Read the model definition and answer for the solid it produces. Units are mm, in the model's axes. Face numbers are marked on the shaded views. A direction names the side the tool comes from. Give positions to 0.01 mm unless a question says otherwise; leave off trailing zeros. Write each loop counter-clockwise with the first axis right and the second up, starting at its lowest first coordinate (ties: lowest second). Pieces come first, ordered by that corner, then holes.
```python
from build123d import *

# Parameters (mm, degrees)
SKETCH011_W         = 30
SKETCH011_H         = 50
PAD009_DEPTH        = 4
SKETCH007_W         = 50
SKETCH007_H         = 25
PAD006_DEPTH        = 4
PAD007_DEPTH        = 3
PAD005_DEPTH        = 1
PAD008_DEPTH        = 3
HOLE001_D           = 4.4
HOLE001_DEPTH       = 25
HOLE001_CSINK_D     = 8
HOLE001_CSINK_ANGLE = 90
SKETCH012_W         = 40.900608
SKETCH012_H         = 56.513194
POCKET_DEPTH        = 25


with BuildPart() as part:
    # Sketch011 → Pad009 (new body)
    with BuildSketch(Plane.XY):
        with Locations((15, 25)):
            Rectangle(SKETCH011_W, SKETCH011_H)
    extrude(amount=PAD009_DEPTH)

    # Sketch007 → Pad006 (join)
    with BuildSketch(Plane(origin=(0, 0, 0), x_dir=(0, -1, 0), z_dir=(-1, 0, 0))):
        with Locations((-25, 16.5)):
            Rectangle(SKETCH007_W, SKETCH007_H)
    extrude(amount=-PAD006_DEPTH)

    # Sketch008 → Pad007 (join)
    with BuildSketch(Plane.XZ):
        Polygon((4, 4), (4, 29), (30, 4), align=None)
    extrude(amount=-PAD007_DEPTH)

    # Sketch009 → Pad005 (join, symmetric)
    with BuildSketch(Plane.XZ.offset(-25)):
        Polygon((4, 4), (4, 29), (30, 4), align=None)
    extrude(amount=PAD005_DEPTH, both=True)

    # Sketch006 → Pad008 (join)
    with BuildSketch(Plane.XZ.offset(-50)):
        Polygon((4, 29), (4, 4), (30, 4), align=None)
    extrude(amount=PAD008_DEPTH)

    # Hole001
    with Locations(Plane.XY.offset(5)):
        with Locations((17, 36.5), (17, 13.5)):
            CounterSinkHole(HOLE001_D / 2, HOLE001_CSINK_D / 2, depth=HOLE001_DEPTH, counter_sink_angle=HOLE001_CSINK_ANGLE)

    # Sketch012 → Pocket (cut)
    with BuildSketch(Plane.XY.offset(13)):
        with Locations((14.816534, 25.266581)):
            Rectangle(SKETCH012_W, SKETCH012_H)
    extrude(amount=POCKET_DEPTH, mode=Mode.SUBTRACT)


solid = part.part
```
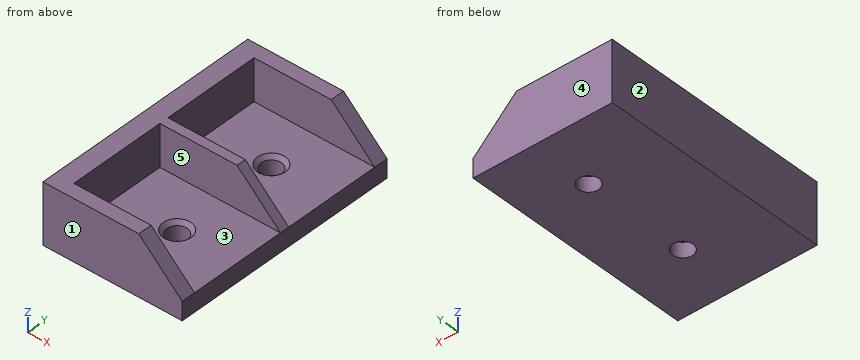
Item 1: Section D-D (y = 23) is taken. Write down the section's boundary in (x, z).
Result set:
outline: (0, 0) - (30, 0) - (30, 4) - (4, 4) - (4, 13) - (0, 13) - close
Item 2: Find the intervals of material crossed by line 1 along Y through (x, z) = (17, 0.8); line 2 along Y through (x, z) = (21, 7.25); line 3 along X through (y, z) = (13.5, 1.65), in increasing order.
Result set:
line 1: y = 0 to 11.3, 15.7 to 34.3, 38.7 to 50
line 2: y = 0 to 3, 24 to 26, 47 to 50
line 3: x = 0 to 14.8, 19.2 to 30
Item 3: Determine the mould class of the marked faces 1, 2 and 3 for opening direction Y: pulls with the +Y half, pulls with the -Y half, needs draft (parallel to the pull), parting line crosses it, or undercut.
Result set:
face 1: pulls with the -Y half
face 2: needs draft
face 3: undercut
Item 4: Each of these flat-tipped pins is pushed along its axis until it touches: pin 1 Ø4 at (x, y) = (17, 36.5) entering from +Z; pin 2 Ø2 at (y, z) = (35, 11) entering from +X; pin 3 Ø5 at (x, y) = (24.5, 37.5) entering from +Z. Where does it stop, or does it pass through?
Result set:
pin 1: passes through
pin 2: stops at x = 4
pin 3: stops at z = 4
Item 5: Section B-B (y = 13.5) is taken. Write down the section's boundary in (x, z), and give its area (3 significant figures).
Result set:
outline: (0, 0) - (14.8, 0) - (14.8, 3.2) - (14, 4) - (4, 4) - (4, 13) - (0, 13) - close; (19.2, 0) - (30, 0) - (30, 4) - (20, 4) - (19.2, 3.2) - close
area: 138 mm2
Item 6: Which of the six approach directions +Z, -Z, +X, -X, +Y, -Y give full straight-line access (tool end or side, diameter ignored) to the marked faces 4 and 5?
Result set:
face 4: +Z, -Z, +X, -X, +Y
face 5: +Z, +X
Item 7: Section C-C (z = 5) is taken. Write down the section's boundary in (x, y).
Result set:
outline: (0, 0) - (28.96, 0) - (28.96, 3) - (4, 3) - (4, 24) - (28.96, 24) - (28.96, 26) - (4, 26) - (4, 47) - (28.96, 47) - (28.96, 50) - (0, 50) - close
Item 8: Section A-A (x = 17) is taken. Write down the section's boundary in (y, z).
Result set:
outline: (0, 0) - (11.3, 0) - (11.3, 3.2) - (10.5, 4) - (3, 4) - (3, 13) - (0, 13) - close; (15.7, 0) - (34.3, 0) - (34.3, 3.2) - (33.5, 4) - (26, 4) - (26, 13) - (24, 13) - (24, 4) - (16.5, 4) - (15.7, 3.2) - close; (38.7, 0) - (50, 0) - (50, 13) - (47, 13) - (47, 4) - (39.5, 4) - (38.7, 3.2) - close
